Answer from the drawing. Dimensions are ordinates in mm from the lowest x, y and z of the part. A direction names the side the tool comes from. Give positions to 0.01 mm unless a question says otherwise; leave off trailing zeros. Order: outer loops, then holes, each group sorted by start corner. A loop starts at its lowest first (then second) coordinate and runs counter-clockwise, first axis right, second up.
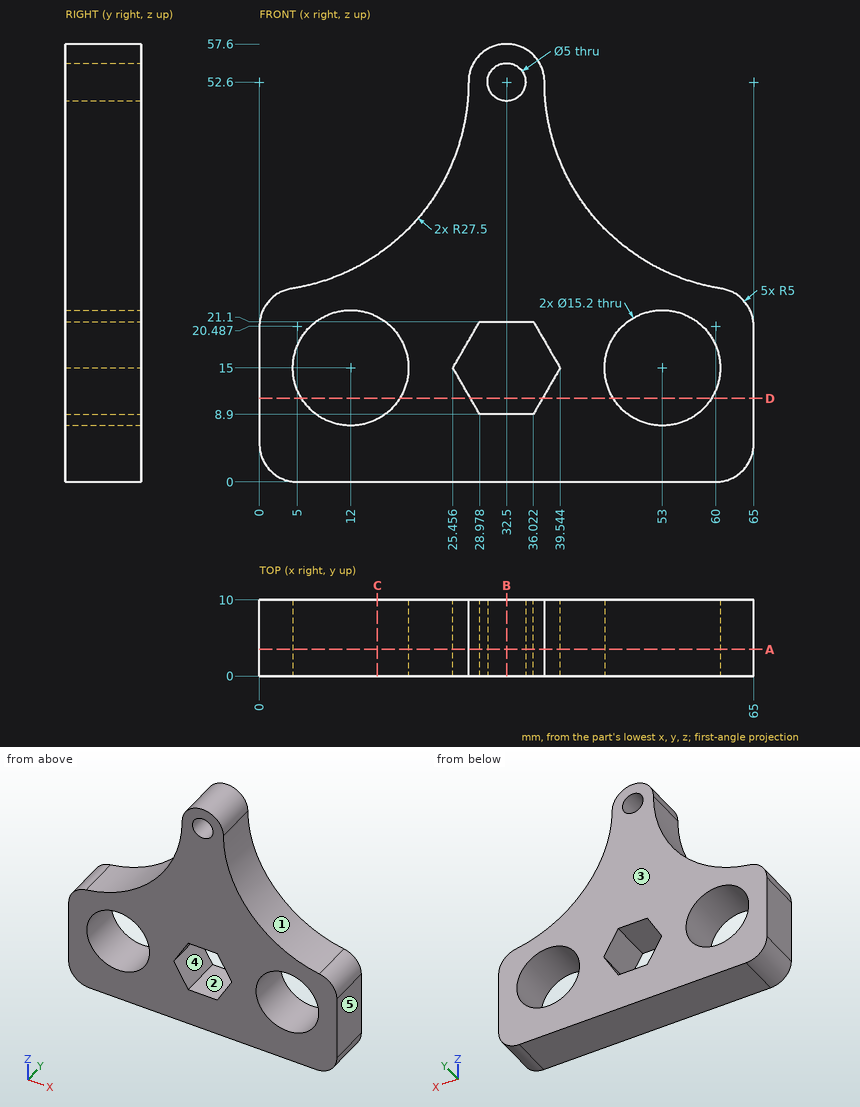
1) The part is cut by section C-C on x = 15.5. Determine the outline of the cut face in (y, z) (1 decimal), and give its area (3 significant figures).
Final values:
outline: (0, 0) - (10, 0) - (10, 8.3) - (0, 8.3) - close; (0, 21.7) - (10, 21.7) - (10, 29.9) - (0, 29.9) - close
area: 164 mm2
2) The part is cut by section A-A on y = 3.5. Determine the outline of the cut face in (x, z), and give its area (3 significant figures).
Final values:
outline: (0, 5) arc R5 ccw to (5, 0) - (60, 0) arc R5 ccw to (65, 5) - (65, 20.49) arc R5 ccw to (60.77, 25.43) arc R27.5 cw to (37.5, 52.6) arc R5 ccw to (27.5, 52.6) arc R27.5 cw to (4.23, 25.43) arc R5 ccw to (0, 20.49) - close; hole circle Ø15.2 at (12, 15); hole (25.46, 15) - (28.98, 8.9) - (36.02, 8.9) - (39.54, 15) - (36.02, 21.1) - (28.98, 21.1) - close; hole circle Ø5 at (32.5, 52.6); hole circle Ø15.2 at (53, 15)
area: 1,740 mm2
3) A tool of negligible diameter and unlimited length cuts with its end or side. For the marked faces 1 and 2, from which of +Z, -Z, +X, -X, +Y, -Y can it reach the whole face along a straight path? Write none if from no direction.
Final values:
face 1: +Z, +X, +Y, -Y
face 2: +Y, -Y
4) The part is cut by section D-D on z = 11. Determine the outline of the cut face in (x, y).
Final values:
outline: (0, 0) - (5.54, 0) - (5.54, 10) - (0, 10) - close; (18.46, 0) - (27.77, 0) - (27.77, 10) - (18.46, 10) - close; (37.23, 0) - (46.54, 0) - (46.54, 10) - (37.23, 10) - close; (59.46, 0) - (65, 0) - (65, 10) - (59.46, 10) - close
5) For a pull along X with two mould halves and no side action, classify the marked faces 3, 4 and 5 as released by +X, released by -X, zero draft, split by the parting line, or undercut.
Final values:
face 3: zero draft
face 4: undercut
face 5: released by +X
6) Given pin 1 (1.5 mm diameter, centred on y = 4.5, z = 47, fed in from +X), flat-ended and moving along its own axis, determine where the tip first touches the part or whether it passes through.
Final values:
pin 1: stops at x = 38.24
7) Consider L1, parallel to Z at x = 34, y = 2.5; L2, parallel to X at y = 4.5, z = 13; L3, parallel to X at y = 8.5, z = 16 (1 decimal). Determine where each line is inside the solid, lowest interval first.
Final values:
L1: z = 0 to 8.9, 21.1 to 50.6, 54.6 to 57.37
L2: x = 0 to 4.67, 19.33 to 26.61, 38.39 to 45.67, 60.33 to 65
L3: x = 0 to 4.5, 19.5 to 26, 39 to 45.5, 60.5 to 65
8) The part is cut by section B-B on x = 32.5. Determine the outline of the cut face in (y, z).
Final values:
outline: (0, 0) - (10, 0) - (10, 8.9) - (0, 8.9) - close; (0, 21.1) - (10, 21.1) - (10, 50.1) - (0, 50.1) - close; (0, 55.1) - (10, 55.1) - (10, 57.6) - (0, 57.6) - close
